Source: three-view drawing plus pictorial views. Frame: mm from the lowest corner of the part. A direction names the side the tool comes from. Coordinates: 2 decimals unless noted, no trailing zeros. Order: outer loops, then holes, each group sorted by start corner. A loop starts at its lowest first (then second) coordinate and runs counter-clockwise, first axis right, second up. Notation, with made-up numbers: M 57,70.5 L 92,70.5 A30 cw 92,99.5 Z; hole C 65,83 d5. An arc over 180 degrees is marked long. One line per question, with ' | ' between items.
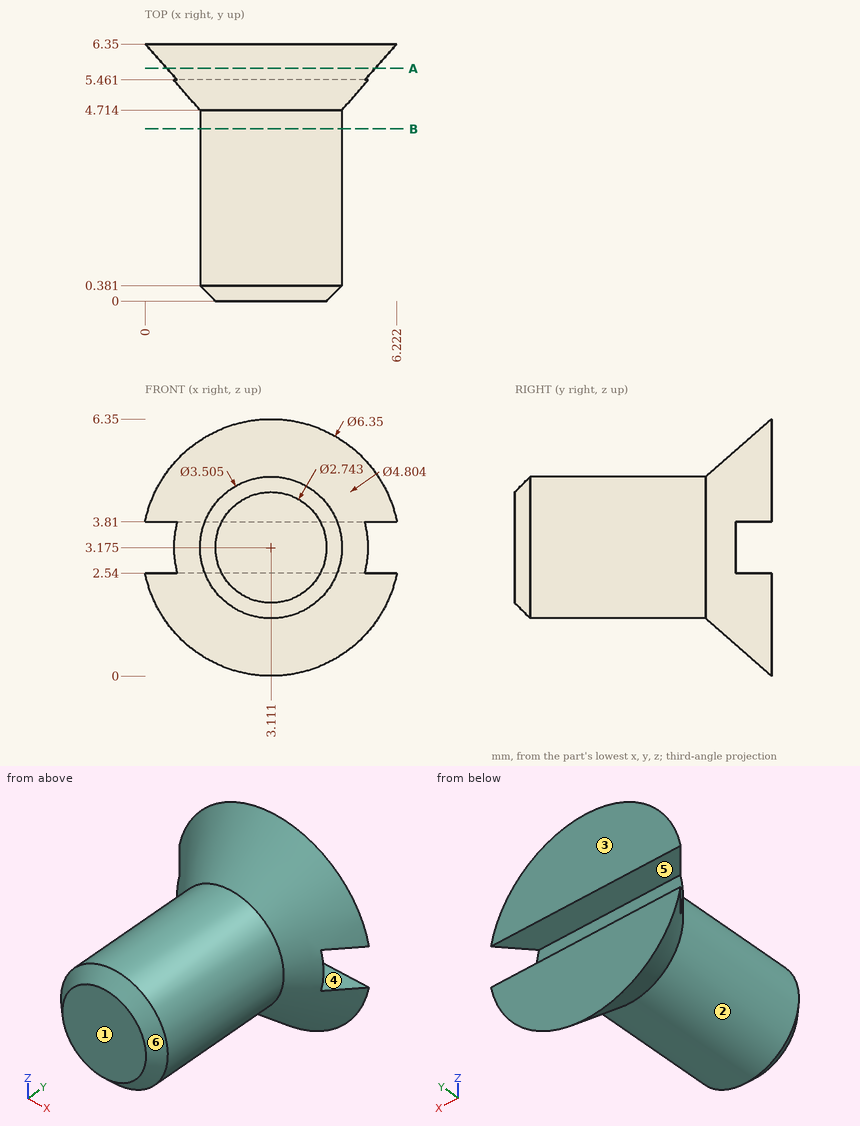
1. Pin query (flat end, axial travel): P1, Ø0.7, axis at x = 4.5, y = 6, coming from the +Z side (1 decimal); P2, Ø1.5, axis at y = 2.5, z = 1.5, coming from the +X side; P3, Ø2, axis at x = 3, y = 3.5, coming from the -Z side. Return the tip coordinate at first contact, or that it passes through.
Response values:
P1: stops at z = 6.1 | P2: stops at x = 4.6 | P3: stops at z = 1.42
2. Section A-A, the plane y = 5.75. Output: boundary loops of the cut face in (x, z) (1 decimal).
Response values:
outline: M 0.5,2.5 A2.7 ccw 5.7,2.5 Z; M 0.5,3.8 L 5.7,3.8 A2.7 ccw Z
3. Material intervals for line 1 (X direction, y = 1, z = 3.25); line 2 (Y direction, x = 3, z = 3.5); line 3 (Z direction, x = 3.5, y = 3.5) (1 decimal), sorted ascending. Write a range as [from, to].
Response values:
line 1: x = [1.36, 4.86] | line 2: y = [0, 5.46] | line 3: z = [1.5, 4.9]
4. Section B-B, the plane y = 4.25. Output: boundary loops of the cut face in (x, z) (1 decimal).
Response values:
outline: C 3.1,3.2 d3.5
5. Access query for the marked faces 1 and 2. Directions: +Z, -Z, +X, -X, +Y, -Y. A direction counts if a zero-diameter tool reaches every point of the face in a straight line with its end or side. Return the directions, or none.
Response values:
face 1: +Z, -Z, +X, -X, -Y | face 2: -Y
6. Draft query along Z for the marked faces 3, 4, 5 and 6. Return one class per face: pulls with the +Z half, pulls with the -Z half, needs draft (parallel to the pull), parting line crosses it, or undercut.
Response values:
face 3: needs draft | face 4: undercut | face 5: undercut | face 6: parting line crosses it
